from build123d import *

# Parameters (mm, degrees)
BOSS_EXTRUDE1_DEPTH = 27.5
SKETCH3_W           = 6.5
SKETCH3_H           = 8.75
CUT_EXTRUDE1_DEPTH  = 5
SKETCH5_R           = 1
CUT_EXTRUDE2_DEPTH  = 232.527578609
SKETCH6_W           = 25.5
SKETCH6_H           = 20
CUT_EXTRUDE3_DEPTH  = 9
SKETCH7_W           = 25.5
SKETCH7_H           = 20
CUT_EXTRUDE4_DEPTH  = 9
SKETCH8_R           = 2.5
SKETCH8_R_2         = 2
BOSS_EXTRUDE2_DEPTH = 2
SKETCH10_W          = 57.691481813
SKETCH10_H          = 15.5
CUT_EXTRUDE5_DEPTH  = 232.800925283


with BuildPart() as part:
    # Sketch1 → Boss-Extrude1 (new body)
    with BuildSketch(Plane.XY):
        with BuildLine():
            Line((-4.499758881, 1.478052726), (0, 1.478052726))
            Line((0, 1.478052726), (4.499758881, 1.478052726))
            Line((4.499758881, 1.478052726), (7.5, -1.917676035))
            Line((7.5, -1.917676035), (14, -1.917676035))
            Line((14, -1.917676035), (14, 0.082323965))
            Line((14, 0.082323965), (8.40173886, 0.082323965))
            Line((8.40173886, 0.082323965), (5.401497741, 3.478052726))
            Line((5.401497741, 3.478052726), (5.401497741, 3.774186429))
            ThreePointArc((5.401497741, 3.774186429), (9.689685466, 14.274523461), (20.102441447, 18.771204977))
            Line((20.102441447, 18.771204977), (106, 20.484092471))
            Line((106, 20.484092471), (191.897558553, 18.771204977))
            ThreePointArc((191.897558553, 18.771204977), (202.310314534, 14.274523461), (206.598502259, 3.774186429))
            Line((206.598502259, 3.774186429), (206.598502259, 3.478052726))
            Line((206.598502259, 3.478052726), (203.59826114, 0.082323965))
            Line((203.59826114, 0.082323965), (198, 0.082323965))
            Line((198, 0.082323965), (198, -1.917676035))
            Line((198, -1.917676035), (204.5, -1.917676035))
            Line((204.5, -1.917676035), (207.500241119, 1.478052726))
            Line((207.500241119, 1.478052726), (212, 1.478052726))
            Line((212, 1.478052726), (216.499758881, 1.478052726))
            Line((216.499758881, 1.478052726), (219.5, -1.917676035))
            Line((219.5, -1.917676035), (226, -1.917676035))
            Line((226, -1.917676035), (226, 0.082323965))
            Line((226, 0.082323965), (220.40173886, 0.082323965))
            Line((220.40173886, 0.082323965), (217.401497741, 3.478052726))
            Line((217.401497741, 3.478052726), (217.401497741, 4.065324402))
            ThreePointArc((217.401497741, 4.065324402), (211.999722772, 17.736162927), (198.712315146, 24.022322116))
            Line((198.712315146, 24.022322116), (120.020833333, 32.082323965))
            ThreePointArc((120.020833333, 32.082323965), (118.430658364, 38.567884851), (114.020833333, 43.582323965))
            Line((114.020833333, 43.582323965), (97.979166667, 43.582323965))
            ThreePointArc((97.979166667, 43.582323965), (93.569341636, 38.567884851), (91.979166667, 32.082323965))
            Line((91.979166667, 32.082323965), (13.287684854, 24.022322116))
            ThreePointArc((13.287684854, 24.022322116), (0.000277228, 17.736162927), (-5.401497741, 4.065324402))
            Line((-5.401497741, 4.065324402), (-5.401497741, 3.478052726))
            Line((-5.401497741, 3.478052726), (-8.40173886, 0.082323965))
            Line((-8.40173886, 0.082323965), (-14, 0.082323965))
            Line((-14, 0.082323965), (-14, -1.917676035))
            Line((-14, -1.917676035), (-7.5, -1.917676035))
            Line((-7.5, -1.917676035), (-4.499758881, 1.478052726))
        make_face()
    extrude(amount=BOSS_EXTRUDE1_DEPTH)

    # Sketch3 → Cut-Extrude1 (cut)
    with BuildSketch(Plane.XZ.offset(1.917676035)):
        with Locations((10.75, 23.125)):
            Rectangle(SKETCH3_W, SKETCH3_H)
        with Locations((10.75, 4.375)):
            Rectangle(SKETCH3_W, SKETCH3_H)
        with Locations((201.25, 4.375)):
            Rectangle(SKETCH3_W, SKETCH3_H)
        with Locations((201.25, 23.125)):
            Rectangle(SKETCH3_W, SKETCH3_H)
    extrude(amount=-CUT_EXTRUDE1_DEPTH, mode=Mode.SUBTRACT)

    # Sketch5 → Cut-Extrude2 (cut, through all)
    with BuildSketch(Plane.XZ.offset(-1.478052726)):
        with Locations(Location((0, 18.75, 0), (0, 0, 270))):
            Circle(SKETCH5_R)
        with Locations(Location((0, 8.75, 0), (0, 0, 270))):
            Circle(SKETCH5_R)
        with Locations(Location((212, 8.75, 0), (0, 0, 270))):
            Circle(SKETCH5_R)
        with Locations(Location((212, 18.75, 0), (0, 0, 270))):
            Circle(SKETCH5_R)
    extrude(amount=-CUT_EXTRUDE2_DEPTH, mode=Mode.SUBTRACT)

    # Sketch6 → Cut-Extrude3 (cut)
    with BuildSketch(Plane.ZY.offset(5.401497741)):
        with Locations((13.75, 14.065324402)):
            Rectangle(SKETCH6_W, SKETCH6_H)
    extrude(amount=-CUT_EXTRUDE3_DEPTH, mode=Mode.SUBTRACT)

    # Sketch7 → Cut-Extrude4 (cut)
    with BuildSketch(Plane(origin=(217.401497741, 0, 0), x_dir=(0, 0, -1), z_dir=(1, 0, 0))):
        with Locations((-13.75, 14.065324402)):
            Rectangle(SKETCH7_W, SKETCH7_H)
    extrude(amount=-CUT_EXTRUDE4_DEPTH, mode=Mode.SUBTRACT)

    # Sketch8 → Boss-Extrude2 (add)
    # profile 1 of 4: a face of its own
    with BuildSketch(Plane(origin=(0, 4.065324402, 0), x_dir=(1, 0, 0), z_dir=(0, 1, 0))):
        with Locations(Location((0, -8.75, 0), (0, 0, 90))):
            Circle(SKETCH8_R)
        with Locations(Location((0, -8.75, 0), (0, 0, 270))):
            Circle(SKETCH8_R_2, mode=Mode.SUBTRACT)
    # profile 2 of 4: a face of its own
    with BuildSketch(Plane(origin=(0, 4.065324402, 0), x_dir=(1, 0, 0), z_dir=(0, 1, 0))):
        with Locations(Location((0, -18.75, 0), (0, 0, 90))):
            Circle(SKETCH8_R)
        with Locations(Location((0, -18.75, 0), (0, 0, 90))):
            Circle(SKETCH8_R_2, mode=Mode.SUBTRACT)
    # profile 3 of 4: a face of its own
    with BuildSketch(Plane(origin=(0, 4.065324402, 0), x_dir=(1, 0, 0), z_dir=(0, 1, 0))):
        with Locations(Location((212, -18.75, 0), (0, 0, 90))):
            Circle(SKETCH8_R)
        with Locations(Location((212, -18.75, 0), (0, 0, 270))):
            Circle(SKETCH8_R_2, mode=Mode.SUBTRACT)
    # profile 4 of 4: a face of its own
    with BuildSketch(Plane(origin=(0, 4.065324402, 0), x_dir=(1, 0, 0), z_dir=(0, 1, 0))):
        with Locations(Location((212, -8.75, 0), (0, 0, 90))):
            Circle(SKETCH8_R)
        with Locations(Location((212, -8.75, 0), (0, 0, 90))):
            Circle(SKETCH8_R_2, mode=Mode.SUBTRACT)
    extrude(amount=BOSS_EXTRUDE2_DEPTH)

    # Sketch10 → Cut-Extrude5 (cut, through all)
    with BuildSketch(Plane(origin=(0, 0, 0), x_dir=(1, 0, 0), z_dir=(0, 1, 0))):
        with Locations((163.86657424, -13.75)):
            Rectangle(SKETCH10_W, SKETCH10_H)
        with Locations((48.133425761, -13.75)):
            Rectangle(SKETCH10_W, SKETCH10_H)
    extrude(amount=CUT_EXTRUDE5_DEPTH, mode=Mode.SUBTRACT)


solid = part.part
Build history of the part. All positions in model axes, mm. A direction names the side the tool comes from. Give positions to 0.01 mm unless a question says otherwise; leave off trailing zeros. Order: outer loops, then holes, each group sorted by start corner. A loop starts at its lowest first (then second) coordinate and runs counter-clockwise, first axis right, second up. Notation, with made-up numbers: M -39.75,42.5 L -35.75,42.5 A18 cw -35.75,51.5 Z; hole C -21,64.25 d1. An arc over 180 degrees is marked long. Use one line per item in the form item = value.
1) Two-plate mould, pull along X, no slides. Class faces 4 (the face through (118.474, 38.484, 13.558)), 5 (the face through (76.979, 25, 14)), 6 (the face through (105, 23, 27.5)): released by +X, released by -X, zero draft, split by the parting line, or undercut.
Calculated:
face_4 = released by +X
face_5 = undercut
face_6 = zero draft
2) Saw through at B-B (y = 11.5). Give the cut face in (x, z), plus the area to 3 significant figures.
Calculated:
outline = M -3.97,0 L 7.54,0 L 7.54,27.5 L -3.97,27.5 L -3.97,26.5 L 3.6,26.5 L 3.6,1 L -3.97,1 Z; M 204.46,0 L 215.97,0 L 215.97,1 L 208.4,1 L 208.4,26.5 L 215.97,26.5 L 215.97,27.5 L 204.46,27.5 Z
area = 247 mm2
3) Saw through at A-A (x = 62). Give the cut face in (y, z), plus the area to 3 significant figures.
Calculated:
outline = M 19.61,0 L 29.01,0 L 29.01,6 L 19.61,6 Z; M 19.61,21.5 L 29.01,21.5 L 29.01,27.5 L 19.61,27.5 Z
area = 113 mm2
4) Probe probe 1 along X at (y, z) = (4.75, 18.75); probe 2 along Z at (x, y) = (46, 25); probe 3 along X at (y, z) = (2.8, 18.75). List the from-to ranges inside material, lowest first.
Calculated:
probe_1 = -2.5 to -2, 2 to 2.5, 3.6 to 5.43, 206.57 to 208.4, 209.5 to 210, 214 to 214.5
probe_2 = 0 to 6, 21.5 to 27.5
probe_3 = -6 to -1, 1 to 6, 206 to 211, 213 to 218
5) Saw through at C-C (x = 37.5). Give the cut face in (y, z), plus the area to 3 significant figures.
Calculated:
outline = M 19.12,0 L 26.5,0 L 26.5,6 L 19.12,6 Z; M 19.12,21.5 L 26.5,21.5 L 26.5,27.5 L 19.12,27.5 Z
area = 88.6 mm2
6) Saw through at D-D (y = 39.5). Give the cut face in (x, z).
Calculated:
outline = M 94.1,0 L 117.9,0 L 117.9,27.5 L 94.1,27.5 Z
7) Tool access for faces 1 (the face through (0, 6.065, 21)), 2 (the face through (212, 10, 26.5)), 3 (the face through (0, 1.478, 14)): list every direction of +Z, -Z, +X, -X, +Y, -Y with a clear straight run to the whole face (end or side of a thin tool).
Calculated:
face_1 = -X, +Y
face_2 = +X, +Y
face_3 = +Z, -Z, -Y
8) Drop flat-ended pins along their axis: pin 1 (4 mm diameter, centred on x = 212, z = 20, fed in from +Y); pin 2 (8 mm diameter, centred on x = 17.5, z = 8.5, fed in from +Y); pin 3 (4 mm diameter, centred on x = 58.5, z = 7.5, fed in from -Y). Give the stop position or say it passes through.
Calculated:
pin_1 = 6.07
pin_2 = 24.77
pin_3 = 19.51
